```python
from build123d import *

# Parameters (mm, degrees)
SKETCH1_R           = 1.5
SKETCH1_R_2         = 3.5
BOSS_EXTRUDE1_DEPTH = 2
FILLET1_R           = 5


with BuildPart() as part:
    # Sketch1 → Boss-Extrude1 (new body)
    with BuildSketch(Plane(origin=(0, 0, 0), x_dir=(0, 0, -1), z_dir=(1, 0, 0))):
        with BuildLine():
            Line((0, 7.5), (12, 7.5))
            Line((12, 7.5), (12, -7.5))
            Line((12, -7.5), (0, -7.5))
            ThreePointArc((0, -7.5), (-7.5, 0), (0, 7.5))
        make_face()
        with Locations((6.905099565, -4)):
            Circle(SKETCH1_R, mode=Mode.SUBTRACT)
        with Locations((6.905099565, 4)):
            Circle(SKETCH1_R, mode=Mode.SUBTRACT)
        Circle(SKETCH1_R_2, mode=Mode.SUBTRACT)
    extrude(amount=BOSS_EXTRUDE1_DEPTH)

    # Fillet1
    fillet1_edges = [part.edges().sort_by_distance(p)[0] for p in [
        (1, 7.5, -12),
        (1, -7.5, -12),
    ]]
    fillet(fillet1_edges, radius=FILLET1_R)


solid = part.part
```
Verification items for the finished model (mm, model axes). Coordinates: 2 decimals unless noted, no trailing zeros. Loops run counter-clockwise (first coordinate to the right, second up) from the corner with the lowest first, then second, coordinate; pieces in that order, holes last. Notation, with made-up numbers: (89.5, 89) - (144.5, 89) arc R18 ccw to (144.5, 122) - close; hole circle Ø8 at (-28, 48.5). An arc over 180 degrees is marked (long way). Return JSON: item names as keys, results as strings.
1. Mould release check, pull along Y, two halves, no side actions. Record for faces 1 (the cylindrical face through (0.986, -2.986, -5.8)), 2 (the flat face through (1, 7.5, -3)), 3 (the flat face through (1, -7.5, -4)), 4 (the flat face through (0, 0, -5)): +Y half, -Y half, draft (parallel to the pull), parting line (faces both ways), or undercut.
Established:
{"face 1": "undercut", "face 2": "+Y half", "face 3": "-Y half", "face 4": "draft"}
2. Section check C-C, the plane z = -2.75. Record the boundary of the cut face in (x, y), then the cut area to 3 significant figures.
Established:
{"outline": "(0, -7.5) - (2, -7.5) - (2, -2.17) - (0, -2.17) - close; (0, 2.17) - (2, 2.17) - (2, 7.5) - (0, 7.5) - close", "area": "21.3 mm2"}
3. Section check B-B, the plane x = 1.3. Record the boundary of the cut face in (y, z), then the cut area to 3 significant figures.
Established:
{"outline": "(-7.5, -7) arc R5 ccw to (-2.5, -12) - (2.5, -12) arc R5 ccw to (7.5, -7) - (7.5, 0) arc R7.5 ccw to (-7.5, 0) - close; hole circle Ø3 at (-4, -6.91); hole circle Ø7 at (0, 0); hole circle Ø3 at (4, -6.91)", "area": "205 mm2"}
4. Go/stop test with a flat-tipped pin: pin 1 (5 mm diameter, centred on y = 4, z = -6.91, fed in from +X). Record where the tip stops, or that it passes through.
Established:
{"pin 1": "stops at x = 2"}
5. Section check A-A, the plane y = 0. Record the boundary of the cut face in (x, z).
Established:
{"outline": "(0, -12) - (2, -12) - (2, -3.5) - (0, -3.5) - close; (0, 3.5) - (2, 3.5) - (2, 7.5) - (0, 7.5) - close"}
6. Thickness scan on L1, parallel to Y at x = 1, z = -7.25; L2, parallel to Y at x = 1.55, z = -6.25; L3, parallel to Y at x = 1.25, z = 2.75. Record the ranges inside material, lowest first.
Established:
{"L1": "y = -7.49 to -5.46, -2.54 to 2.54, 5.46 to 7.49", "L2": "y = -7.5 to -5.35, -2.65 to 2.65, 5.35 to 7.5", "L3": "y = -6.98 to -2.17, 2.17 to 6.98"}
